```python
from build123d import *

# Parameters (mm, degrees)
F0_W     = 1300
F0_H     = 600
F1_DEPTH = 1200
F2_W     = 1500
F2_H     = 1147.1251249313
F2_W_2   = 1300
F2_H_2   = 600
F3_DEPTH = 25


with BuildPart() as f1:
    # F0 (on Front) → F1 (new body)
    with BuildSketch(Plane.XZ):
        with Locations((650, 300)):
            Rectangle(F0_W, F0_H)
    extrude(amount=F1_DEPTH)

    # F2 (on face) → F3 (join)
    with BuildSketch(Plane.XZ.offset(1200)):
        with Locations((676.4374375343, 500)):
            Rectangle(F2_W, F2_H)
        with Locations((650, 300)):
            Rectangle(F2_W_2, F2_H_2, mode=Mode.SUBTRACT)
        with Locations((650, 300)):
            Rectangle(F2_W_2, F2_H_2)
    extrude(amount=F3_DEPTH)


solid = f1.part
```
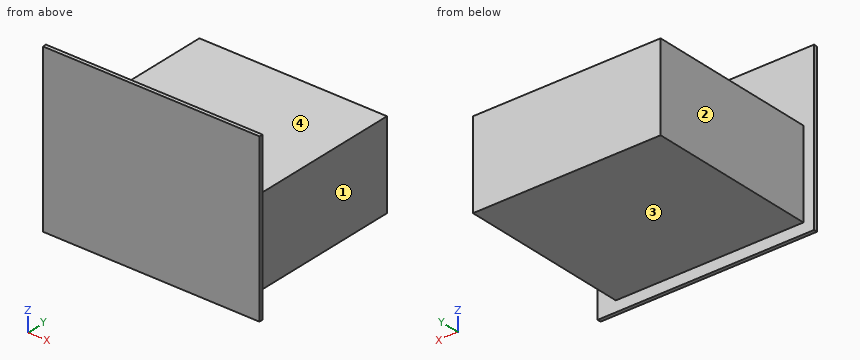
Input: part model. Units: mm. Frame: model coordinates. Face numbers are marked on the shaded views. A direction names the side the tool comes from. Round coordinates to 2 decimals unless told otherwise and drop trailing zeros. Loops run counter-clockwise (first coordinate to the right, second up) from the corner with the lowest first, then second, coordinate; pieces in that order, holes last. Notation, with made-up numbers: (-12, 64.25) -> (17, 64.25) arc R10 ccw to (17, 72.25) -> close; hole circle Ø6 at (-28.75, -4.5). An arc over 180 degrees is marked (long way). Use one line per item in the form item = value. Start each with the question number.
Item 1: Section query B-B on x = 1269.5. Return the cut outline in (y, z).
Item 2: Section query D-D on z = 938.5. Return the cut outline in (x, y), then the cut area to 3 significant figures.
Item 3: Section query A-A on z = 69. Return the cut outline in (x, y).
Item 4: Contact query for flat-ended pins moving along their axis: pin 1 Ø8 at (x, y) = (428, -606) entering from +Z; pin 2 Ø1.5 at (y, z) = (-707, 490) entering from +X; pin 3 Ø6 at (x, y) = (878.5, -869) entering from -Z. Output: stop coordinate, or through.
Item 5: Set-up query: the marked faces 1, 2, 3 and 4. Return all of +Z, -Z, +X, -X, +Y, -Y with unobstructed straight access to the full face (end or side cutting, diameter ignored); none if empty.
Item 6: Material intervals for L1, parallel to Z at x = 159, y = -527; L2, parallel to X at y = -770.5, z = 423; L3, parallel to Y at x = 433, z = 910, sorted ascending. Write a range as from..to.
Item 7: Section query C-C on y = -363.5. Return the cut outline in (x, z), then the cut area to 3 significant figures.
Ans:
q1.outline = (-1225, -73.56) -> (-1200, -73.56) -> (-1200, 0) -> (0, 0) -> (0, 600) -> (-1200, 600) -> (-1200, 1073.56) -> (-1225, 1073.56) -> close
q2.outline = (-73.56, -1225) -> (1426.44, -1225) -> (1426.44, -1200) -> (-73.56, -1200) -> close
q2.area = 37,500 mm^2
q3.outline = (-73.56, -1225) -> (1426.44, -1225) -> (1426.44, -1200) -> (1300, -1200) -> (1300, 0) -> (0, 0) -> (0, -1200) -> (-73.56, -1200) -> close
q4.pin_1 = 600
q4.pin_2 = 1300
q4.pin_3 = 0
q5.face_1 = +Z, -Z, +X, +Y
q5.face_2 = +Z, -Z, -X, +Y
q5.face_3 = -Z, +X, -X, +Y
q5.face_4 = +Z, +X, -X, +Y
q6.L1 = 0..600
q6.L2 = 0..1300
q6.L3 = -1225..-1200
q7.outline = (0, 0) -> (1300, 0) -> (1300, 600) -> (0, 600) -> close
q7.area = 780,000 mm^2
